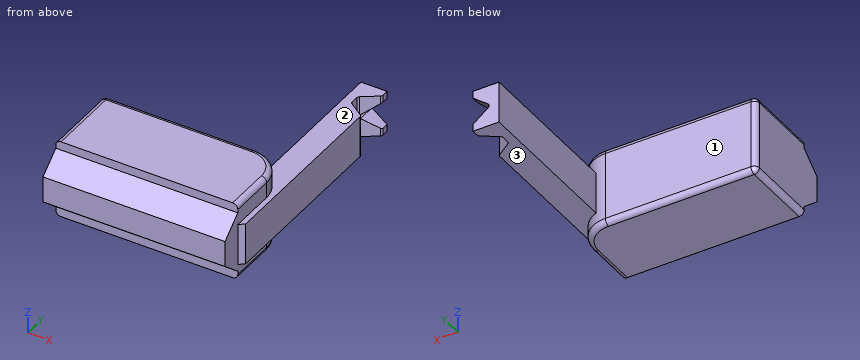
from build123d import *

# Parameters (mm, degrees)
BOSS_EXTRU_1_DEPTH      = 15
ESQUISSE2_W             = 5
ESQUISSE2_H             = 8
BOSS_EXTRU_2_DEPTH      = 45
ENL_V_MAT_EXTRU_1_DEPTH = 59.864250611
CONG_1_R                = 0.5
ENL_V_MAT_EXTRU_2_DEPTH = 5
BOSS_EXTRU_4_DEPTH      = 35
CONG_3_R                = 1
D_POUILLE2_ANGLE        = 40


with BuildPart() as part:
    # Esquisse1 → Boss.-Extru.1 (new body)
    with BuildSketch(Plane.XY):
        with BuildLine():
            Line((0, 0), (35, 0))
            Line((35, 0), (35, 9))
            ThreePointArc((35, 9), (33.242640687, 13.242640687), (29, 15))
            Line((29, 15), (0, 15))
            Line((0, 15), (0, 0))
        make_face()
    extrude(amount=BOSS_EXTRU_1_DEPTH)

    # Esquisse2 → Boss.-Extru.2 (add)
    with BuildSketch(Plane.XZ):
        with Locations((33.5, 7)):
            Rectangle(ESQUISSE2_W, ESQUISSE2_H)
    extrude(amount=-BOSS_EXTRU_2_DEPTH)

    # Esquisse3 → Enlèv. mat.-Extru.1 (cut, through all)
    with BuildSketch(Plane(origin=(0, 0, 3), x_dir=(-1, 0, 0), z_dir=(0, 0, -1))):
        Polygon((-36, 43.455794604), (-36, 36.867183113), (-32.723391823, 39.161488859), (-32.723391823, 41.161488859), align=None)
    extrude(amount=-ENL_V_MAT_EXTRU_1_DEPTH, mode=Mode.SUBTRACT)

    # Congé1
    cong_1_edges = [part.edges().sort_by_distance(p)[0] for p in [
        (36, 36.867183113, 7),
        (36, 43.455794604, 7),
        (32.723391823, 41.161488859, 7),
        (32.723391823, 39.161488859, 7),
    ]]
    fillet(cong_1_edges, radius=CONG_1_R)

    # Esquisse4 → Enlèv. mat.-Extru.2 (cut)
    with BuildSketch(Plane(origin=(0, 45, 0), x_dir=(1, 0, 0), z_dir=(0, 1, 0))):
        with BuildLine():
            Line((36, -4.374713624), (33.095619285, -6.60332333))
            ThreePointArc((33.095619285, -6.60332333), (32.9, -7), (33.095619285, -7.39667667))
            Line((33.095619285, -7.39667667), (36, -9.625286376))
            Line((36, -9.625286376), (36, -4.374713624))
        make_face()
    extrude(amount=-ENL_V_MAT_EXTRU_2_DEPTH, mode=Mode.SUBTRACT)

    # Esquisse6 → Boss.-Extru.4 (add)
    with BuildSketch(Plane.ZY):
        Polygon((13.356398525, 0), (1.643601475, 0), (5, -4), (10, -4), align=None)
    extrude(amount=-BOSS_EXTRU_4_DEPTH)

    # Congé3
    cong_3_edges = [part.edges().sort_by_distance(p)[0] for p in [
        (35, 4.5, 0),
        (33.242640687, 13.242640687, 0),
        (14.5, 15, 0),
        (35, 4.5, 15),
        (33.242640687, 13.242640687, 15),
        (14.5, 15, 15),
        (0, 15, 7.5),
        (0, 7.5, 15),
        (0, 7.5, 0),
    ]]
    fillet(cong_3_edges, radius=CONG_3_R)

    # Dépouille2
    d_pouille2_faces = [part.faces().sort_by_distance(p)[0] for p in [
        (35.5, 0, 7),
    ]]
    draft(d_pouille2_faces, Plane(origin=(35, 0, 15), x_dir=(0, 0, 1), z_dir=(1, 0, 0)), D_POUILLE2_ANGLE)


solid = part.part
Read the model definition and answer for the solid it produces. Units are mm, in the model's axes. Face numbers are marked on the shaded views. A direction names the side the tool comes from. Round coordinates to 2 decimals unless told otherwise and drop trailing zeros. Loops run counter-clockwise (first coordinate to the right, second up) from the corner with the lowest first, then second, coordinate; pieces in that order, holes last. Notation, with made-up numbers: (-25, 63) - (-3, 63) arc R8 cw to (-3, 71) - close; hole circle Ø7 at (20, -1). An arc over 180 degrees is marked (long way). One line per question, with ' | ' between items. Start each with the question number.
Q1. Section A-A on x = 4 is taken. Give the vertices of the cut face in (y, z), plus the area to 3 significant figures.
Q2. Flat-ended cylindrical pins translate along their axes: pin 1 (4 mm diameter, centred on y = 27.5, z = 5.5, fed in from -X); pin 2 (5 mm diameter, centred on x = 13.5, z = 2, fed in from +Y); pin 3 (1.3 mm diameter, centred on x = 20.5, z = 14.5, fed in from -Y). Find the tip coordinate at first contact, or state that the pin passes through.
Q3. For the marked faces 1, 2 and 3, determine the directions among +Z, -Z, +X, -X, +Y, -Y from which every point of the face is accessible in a straight line to the end or side of a thin tool.
Q4. Section C-C on y = 29.5 is taken. Give the vertices of the cut face in (x, z), plus the area to 3 significant figures.
Q5. Section D-D on y = 40 is taken. Give the vertices of the cut face in (x, z), plus the area to 3 significant figures.
Q6. Find the intervals of material crossed by L1, parallel to Y at x = 15, z = 7; L2, parallel to Y at x = 7.5, z = 1.25; L3, parallel to X at y = 34, z = 8, in increasing order.
Q7. Section B-B on z = 8 is taken. Give the vertices of the cut face in (x, y).
Established:
1) outline: (-4, 5) - (0, 1.64) - (0, 0) - (14, 0) arc R1 ccw to (15, 1) - (15, 14) arc R1 ccw to (14, 15) - (0, 15) - (0, 13.36) - (-4, 10) - close | area: 258 mm²
2) pin 1: x = 31 | pin 2: y = 15 | pin 3: y = 0
3) face 1: +Z, -Z, -X, +Y | face 2: +Z, +X, +Y | face 3: -Z, +X, +Y
4) outline: (31, 3) - (36, 3) - (36, 11) - (31, 11) - close | area: 40.0 mm²
5) outline: (31, 3) - (32.72, 3) - (32.72, 11) - (31, 11) - close | area: 13.8 mm²
6) L1: -4 to 15 | L2: 0 to 15 | L3: 31 to 36
7) outline: (0, -4) - (35, -4) - (35, 0) - (36, 0.84) - (36, 36.61) arc R0.5 ccw to (35.79, 37.02) - (32.94, 39.01) arc R0.5 cw to (32.72, 39.42) - (32.72, 40.9) arc R0.5 cw to (32.94, 41.31) - (33.88, 41.97) - (33.88, 45) - (31, 45) - (31, 14.66) arc R6 ccw to (29, 15) - (1, 15) arc R1 ccw to (0, 14) - close
